Read the model definition and answer for the solid it produces. Units are mm, in the model's axes. Face numbers are marked on the shaded views. Coordinates: 2 decimals unless noted, no trailing zeros. Loops run counter-clockwise (first coordinate to the right, second up) from the corner with the lowest first, then second, coordinate; pieces in that order, holes last. Notation, with made-up numbers: (38, 30.25) -> (88, 30.25) arc R16 cw to (88, 54.25) -> close; hole circle Ø7 at (39, 37.5). An arc over 180 degrees is marked (long way). Answer as CSV lines item,"result".
```python
from build123d import *

# Parameters (mm, degrees)
F0_R     = 10
F1_DEPTH = 5
F0_R_2   = 12.5
F2_DEPTH = 30
F4_R     = 1


# Not quite as in the source:
# - a fillet or chamfer that OpenCascade refuses, or shapes differently, is made with other operations: its cross-section is extruded or revolved along the edge and cut away or added


with BuildPart() as f1:
    # F0 (on Top) → F1 (new body)
    with BuildSketch(Plane.XY):
        Circle(F0_R)
    extrude(amount=F1_DEPTH)

    # F0 (on Top) → F2 (join)
    with BuildSketch(Plane.XY):
        Circle(F0_R_2)
        Circle(F0_R, mode=Mode.SUBTRACT)
    extrude(amount=F2_DEPTH)

    # F3: fillet of radius 3 on 1 edges, made by hand

    # F3_s1 → F3_t2 (revolve, cut)
    with BuildSketch(Plane.XZ):
        with BuildLine():
            ThreePointArc((12.5, 30), (10.7087121525, 28.9784517816), (10, 27.0419601084))
            Line((10, 27.0419601084), (10, 30))
            Line((10, 30), (12.5, 30))
        make_face()
    revolve(axis=Axis((0, 0, 30), (0, 0, 1)), mode=Mode.SUBTRACT)

    # F4
    f4_edges = [f1.edges().sort_by_distance(p)[0] for p in [
        (-12.5, 0, 30),
    ]]
    fillet(f4_edges, radius=F4_R)


solid = f1.part
```
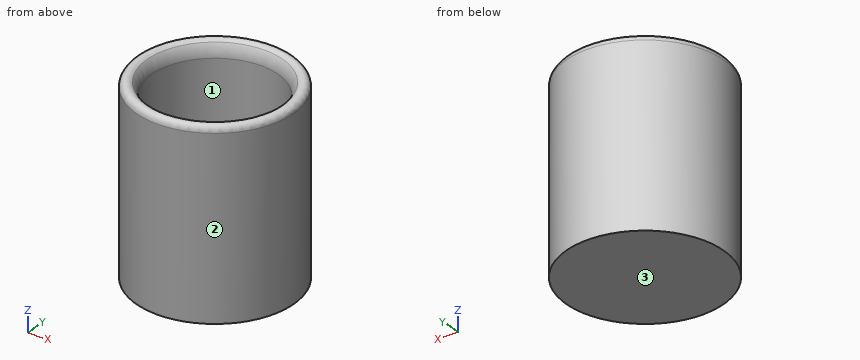
Q1. Find the intervals of material crossed by probe 1 along Y at (x, z) = (0, 20.75); probe 2 along Y at (x, z) = (-1.5, 19.5); probe 3 along Z at (x, y) = (-9.75, 6), in increasing order. Write a range as [from, to].
Results:
probe 1,"y = [-12.5, -10], [10, 12.5]"
probe 2,"y = [-12.41, -9.89], [9.89, 12.41]"
probe 3,"z = [0, 29.36]"
Q2. A cutting plane is placed at A-A, the plane z = 25. Write down the section's boundary in (x, y).
Results:
outline,"circle Ø25 at (0, 0); hole circle Ø20 at (0, 0)"
Q3. For a pull along Y with two mould halves and no side action, classify the marked faces 1, 2 and 3 as pulls with the +Y half, pulls with the -Y half, needs draft (parallel to the pull), parting line crosses it, or undercut.
Results:
face 1,"undercut"
face 2,"parting line crosses it"
face 3,"needs draft"
Q4. Given pin 1 Ø10 at (x, z) = (6.5, 4.5) entering from +Y; pin 2 Ø8 at (x, z) = (9.5, 4.5) entering from -Y (3 decimals); pin 3 Ø4 at (y, z) = (3, 18) entering from -X, each flat-ended and moving along its own axis, determine where each tip first touches the part or whether it passes through.
Results:
pin 1,"stops at y = 12.41"
pin 2,"stops at y = -11.225"
pin 3,"stops at x = -12.46"
